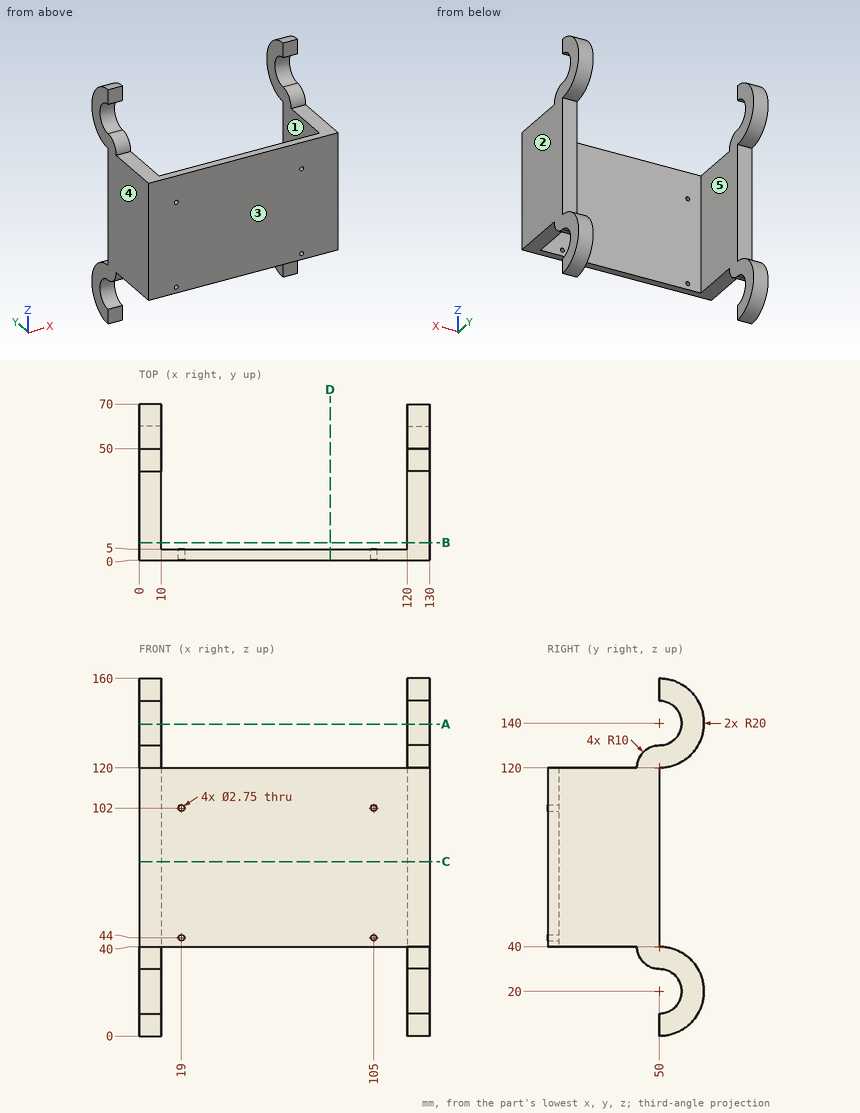
For this review, use the dimensioned drawing (mm, ordinates from the lowest corner) and the shaded views. A direction names the side the tool comes from. Round coordinates to 2 decimals unless told otherwise and drop trailing zeros. Write each loop counter-clockwise with the first axis right and the second up, starting at its lowest first coordinate (ties: lowest second). Pieces come first, ordered by that corner, then holes. Notation, with made-up numbers: (38, 64) - (74, 64) arc R15 cw to (74, 81) - close; hole circle Ø9 at (54, 84.25). An arc over 180 degrees is marked (long way). Answer as CSV lines item,"result". Start each with the question number.
(1) For the marked faces 4 and 5, list the 3-axis set-ups (+Z, -Z, +X, -X, +Y, -Y) from which the entire face can be reached by the end or side of a thin tool; tool diameter is ignored.
(2) We need section B-B on y = 8. State the section outline as (x, z) points, plus the area to 3 significant figures.
(3) We need section C-C on z = 78. State the section outline as (x, y) points, plus the area to 3 significant figures.
(4) To check wall thickness, follow line 1 (Z direction, x = 105, y = 2.65) (3 decimals); line 2 (X direction, y = 3.5, z = 102) (3 decimals); line 3 (X direction, y = 58, z = 29.5). State the ranges of each line that lie inside material, in increasing order.
(5) For pin 1 Ø11 at (x, z) = (126.5, 6.5) entering from -Y; pin 2 Ø1 at (x, z) = (83, 58.5) entering from +Y; pin 3 Ø5 at (x, z) = (4.5, 88) entering from +Y; pin 4 Ø2.5 at (x, z) = (105, 44) entering from -Y, all flat-tipped, find the tip position at first contact; note any pin that passes through.
(6) We need section A-A on z = 139.5. State the section outline as (x, y) points.
(7) Draft analysis for pull direction X (two halves, no side actions). For the marked faces 1, 2 and 3, state which applies: pulls with the +X half, pulls with the -X half, needs draft (parallel to the pull), parting line crosses it, or undercut.
(8) We need section D-D on x = 85.5. State the section outline as (y, z) points, plus the area to 3 significant figures.
Worked answers:
1,face 4,"+Z, -Z, -X, +Y, -Y"
1,face 5,"+Z, -Z, +Y"
2,outline,"(0, 40) - (10, 40) - (10, 120) - (0, 120) - close; (120, 40) - (130, 40) - (130, 120) - (120, 120) - close"
2,area,"1,600 mm²"
3,outline,"(0, 0) - (130, 0) - (130, 50) - (120, 50) - (120, 5) - (10, 5) - (10, 50) - (0, 50) - close"
3,area,"1,550 mm²"
4,line 1,"40 to 42.625, 45.375 to 100.625, 103.375 to 120"
4,line 2,"0 to 17.625, 20.375 to 103.625, 106.375 to 130"
4,line 3,"0 to 10, 120 to 130"
5,pin 1,"y = 50"
5,pin 2,"y = 5"
5,pin 3,"y = 50"
5,pin 4,"through"
6,outline,"(0, 59.99) - (10, 59.99) - (10, 69.99) - (0, 69.99) - close; (120, 59.99) - (130, 59.99) - (130, 69.99) - (120, 69.99) - close"
7,face 1,"undercut"
7,face 2,"pulls with the +X half"
7,face 3,"needs draft"
8,outline,"(0, 40) - (5, 40) - (5, 120) - (0, 120) - close"
8,area,"400 mm²"
